Model file for the job. Use its own axes, mm. Give positions to 0.01 mm unless a question says otherwise; leave off trailing zeros. Loops run counter-clockwise (first coordinate to the right, second up) from the corner with the lowest first, then second, coordinate; pieces in that order, holes last. Notation, with made-up numbers: (20, -5.75) - (25, -5.75) arc R22 cw to (25, 13.25) - close; hole circle Ø10 at (-13.5, 77.25). An arc over 180 degrees is marked (long way). Use a Markdown table: item, result.
from build123d import *

# Parameters (mm, degrees)
CROQUIS1_W              = 300
CROQUIS1_H              = 300
SALIENTE_EXTRUIR1_DEPTH = 3
CROQUIS2_W              = 125
CROQUIS2_H              = 10
CORTAR_EXTRUIR1_DEPTH   = 10


with BuildPart() as part:
    # Croquis1 → Saliente-Extruir1 (new body)
    with BuildSketch(Plane.XY):
        with Locations((150, 150)):
            Rectangle(CROQUIS1_W, CROQUIS1_H)
    extrude(amount=SALIENTE_EXTRUIR1_DEPTH)

    # Croquis2 → Cortar-Extruir1 (cut)
    with BuildSketch(Plane.XY.offset(3)):
        with Locations((82.5, 25)):
            Rectangle(CROQUIS2_W, CROQUIS2_H)
        with Locations((82.5, 165)):
            Rectangle(CROQUIS2_W, CROQUIS2_H)
        with Locations((82.5, 145)):
            Rectangle(CROQUIS2_W, CROQUIS2_H)
        with Locations((82.5, 125)):
            Rectangle(CROQUIS2_W, CROQUIS2_H)
        with Locations((82.5, 105)):
            Rectangle(CROQUIS2_W, CROQUIS2_H)
        with Locations((82.5, 85)):
            Rectangle(CROQUIS2_W, CROQUIS2_H)
        with Locations((82.5, 65)):
            Rectangle(CROQUIS2_W, CROQUIS2_H)
        with Locations((82.5, 45)):
            Rectangle(CROQUIS2_W, CROQUIS2_H)
        with Locations((217.5, 25)):
            Rectangle(CROQUIS2_W, CROQUIS2_H)
        with Locations((217.5, 45)):
            Rectangle(CROQUIS2_W, CROQUIS2_H)
        with Locations((217.5, 65)):
            Rectangle(CROQUIS2_W, CROQUIS2_H)
        with Locations((217.5, 85)):
            Rectangle(CROQUIS2_W, CROQUIS2_H)
        with Locations((217.5, 105)):
            Rectangle(CROQUIS2_W, CROQUIS2_H)
        with Locations((217.5, 125)):
            Rectangle(CROQUIS2_W, CROQUIS2_H)
        with Locations((217.5, 145)):
            Rectangle(CROQUIS2_W, CROQUIS2_H)
        with Locations((217.5, 165)):
            Rectangle(CROQUIS2_W, CROQUIS2_H)
    extrude(amount=-CORTAR_EXTRUIR1_DEPTH, mode=Mode.SUBTRACT)


solid = part.part
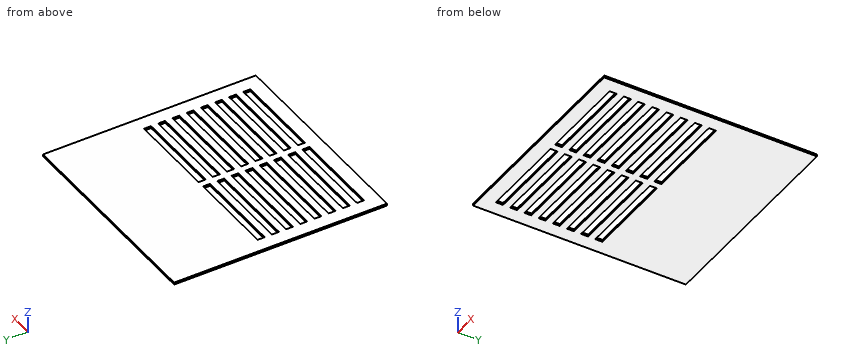
(1) Slice it at B-B, the plane x = 219. Count the separate pieces of the cut face and the enclosed holes in it, plus the area to 3 significant figures.
Computed:
| item | result |
|---|---|
| separate pieces | 9 |
| enclosed holes | 0 |
| area | 660 mm² |
(2) Drill centre line: probe 1 along X at (y, z) = (60.5, 2.75). Where is it in solid material? Low to high. Write a range as [from, to].
Computed:
| item | result |
|---|---|
| probe 1 | [0, 20], [145, 155], [280, 300] |
(3) Slice it at A-A, the plane y = 46.5. Write the cut outline in (x, z), plus the area to 3 significant figures.
Computed:
| item | result |
|---|---|
| outline | (0, 0) - (20, 0) - (20, 3) - (0, 3) - close; (145, 0) - (155, 0) - (155, 3) - (145, 3) - close; (280, 0) - (300, 0) - (300, 3) - (280, 3) - close |
| area | 150 mm² |
